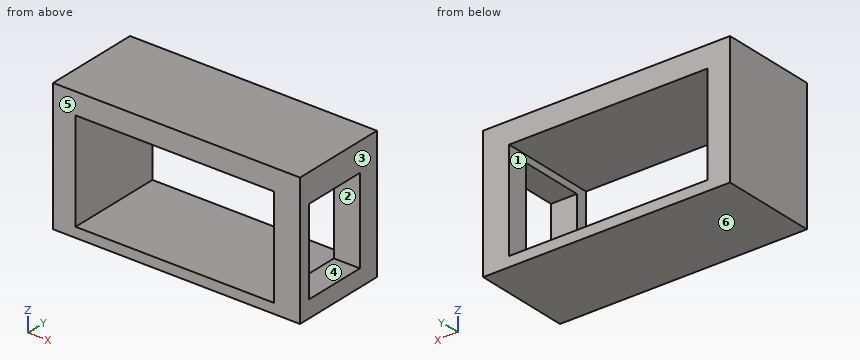
Autodesk Inventor part; units mm, degrees
ref_plane "YZ Plane" through (0, 0, 0) normal (1, 0, 0) x (0, 1, 0)
ref_plane "XZ Plane" through (0, 0, 0) normal (0, 1, 0) x (-1, 0, 0)
ref_plane "XY Plane" through (0, 0, 0) normal (0, 0, 1) x (1, 0, 0)
sketch "Sketch1" plane through (0, 0, 0) normal (1, 0, 0) x (0, 1, 0)
  line L0 (0, 0) -> (-21.59, 0)
  line L1 (-21.59, 0) -> (-21.59, -29.21)
  line L2 (-21.59, -29.21) -> (0, -29.21)
  line L3 (0, -29.21) -> (0, 0)
  dimension "d25" = 29.21
  dimension "d26" = 21.59
extrude "Extrusion1" add sketch "Sketch1" along normal blind 55
sketch "Sketch3" plane through (0, 0, 0) normal (0, 1, 0) x (1, 0, 0)
  line L0 (55, 26.9875) -> (5, 26.9875)
  line L1 (55, 4.7625) -> (5, 4.7625)
  line L2 (49.2125, 26.9875) -> (5, 26.9875)
  line L3 (5, 26.9875) -> (5, 4.7625)
  line L4 (5, 4.7625) -> (49.2125, 4.7625)
  line L5 (49.2125, 4.7625) -> (49.2125, 26.9875)
  point P0 (0, 0)
extrude "Extrusion3" cut sketch "Sketch3" against normal blind 25
sketch "Sketch4" plane through (55, 0, 0) normal (1, 0, 0) x (0, 0, -1)
  line L0 (25.4, -19.05) -> (6.35, -19.05)
  line L1 (6.35, -19.05) -> (6.35, -4.7625)
  line L2 (6.35, -4.7625) -> (25.4, -4.7625)
  line L3 (25.4, -4.7625) -> (25.4, -19.05)
  point P0 (0, 0)
extrude "Extrusion4" cut sketch "Sketch4" against normal blind 25
The listing builds one solid part. Answer for the finished solid, in the listing's coordinates (mm). Face numbers are marked on the shaded views. A direction names the side the tool comes from. Coordinates: 2 decimals unless noted, no trailing zeros. Write each loop counter-clockwise with the first axis right and the second up, starting at its lowest first coordinate (ties: lowest second). Pieces come first, ordered by that corner, then holes. Notation, with made-up numbers: M 23,13 L 59,13 A8 ccw 59,19 Z; hole C -23.5,-13 d1. An arc over 180 degrees is marked long. Write each question's results on one line, items separated by ' | '.
Item 1: The part is cut by section C-C on y = -2.5. Determine the outline of the cut face in (x, z).
Answer below:
outline: M 0,-29.21 L 55,-29.21 L 55,0 L 0,0 Z; hole M 5,-26.99 L 49.21,-26.99 L 49.21,-4.76 L 5,-4.76 Z
Item 2: Consider probe 1 along Z at (x, y) = (24, -4); probe 2 along Z at (x, y) = (53, -14.5); probe 3 along X at (y, z) = (-0.75, -7.25). Determine where each line is inside the solid, lowest interval first. Write a range as [from, to].
Answer below:
probe 1: [-29.21, -26.99], [-4.76, 0] | probe 2: [-29.21, -25.4], [-6.35, 0] | probe 3: [0, 5], [49.21, 55]
Item 3: The part is cut by section D-D on y = -17.25. Determine the outline of the cut face in (x, z).
Answer below:
outline: M 0,-29.21 L 55,-29.21 L 55,-25.4 L 49.21,-25.4 L 49.21,-26.99 L 5,-26.99 L 5,-4.76 L 49.21,-4.76 L 49.21,-6.35 L 55,-6.35 L 55,0 L 0,0 Z
Item 4: For a pull along Y with two mould halves and no side action, classify the marked faces 4, 5 and 6 as released by +Y, released by -Y, zero draft, split by the parting line, or undercut.
Answer below:
face 4: undercut | face 5: released by -Y | face 6: zero draft
Item 5: The part is cut by section A-A on x = 25. Determine the outline of the cut face in (y, z), and give its area (3 significant figures).
Answer below:
outline: M -21.59,-29.21 L 0,-29.21 L 0,-26.99 L -21.59,-26.99 Z; M -21.59,-4.76 L 0,-4.76 L 0,0 L -21.59,0 Z | area: 151 mm2
Item 6: Given P1, Ø12, axis at x = 12.5, z = -11.5, coming from the -Y side, flat-ended and moving along its own axis, determine where the tip first touches the part or whether it passes through.
Answer below:
P1: through
Item 7: Which of the six approach directions +Z, -Z, +X, -X, +Y, -Y give full straight-line access (tool end or side, diameter ignored) to the marked faces 1, 2 and 3?
Answer below:
face 1: +Y, -Y | face 2: +X | face 3: +Z, -Z, +X, +Y, -Y
Item 8: The part is cut by section B-B on z = -21.5. Determine the outline of the cut face in (x, y).
Answer below:
outline: M 0,-21.59 L 5,-21.59 L 5,0 L 0,0 Z; M 49.21,-21.59 L 55,-21.59 L 55,-19.05 L 49.21,-19.05 Z; M 49.21,-4.76 L 55,-4.76 L 55,0 L 49.21,0 Z
